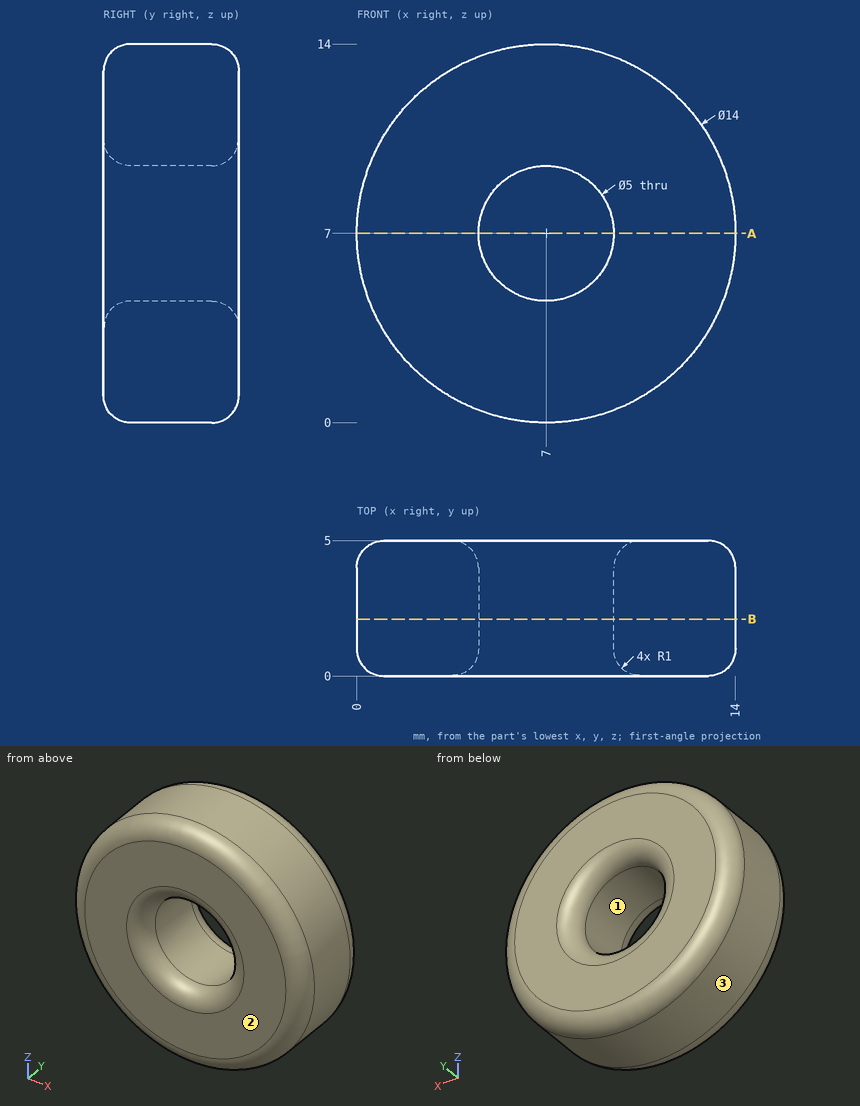
For this review, use the dimensioned drawing (mm, ordinates from the lowest corner) and the shaded views. Give positions to 0.01 mm unless a question says otherwise; leave off trailing zeros. Order: outer loops, then holes, each group sorted by start corner. A loop starts at its lowest first (then second) coordinate and runs counter-clockwise, first axis right, second up.
1) Take a section at A-A (z = 7). Give the boundary of the cut face in (x, y).
2) Wall thickness on line 1 (Z direction, x = 7, y = 2.6); line 2 (Z direction, x = 8, y = 3.75): over which ranges is each line inside the solid? List them lowest first.
3) Insertion check: pin 1 (6.5 mm diameter, centred on x = 7, z = 7, fed in from -Y); pin 2 (1.5 mm diameter, centred on x = 1.5, y = 4, fed in from -Z); pin 3 (3 mm diameter, centred on x = 8.5, y = 3, fed in from -Z); pin 4 (3 mm diameter, centred on x = 9.5, y = 2, fed in from +Z). Each pin has a flat end and moves straight along its axis. Give the tip position at first contact, or say it passes through.
4) Take a section at B-B (y = 2.1). Give the boundary of the cut face in (x, z), then the cut area to 3 significant figures.
5) The part is to be moulded in two halves that separate along X. For the marked faces 1, 2 and 3, say which applies: released by +X, released by -X, zero draft, split by the parting line, or undercut.
Derived:
1. outline: (0, 1) arc R1 ccw to (1, 0) - (3.5, 0) arc R1 ccw to (4.5, 1) - (4.5, 4) arc R1 ccw to (3.5, 5) - (1, 5) arc R1 ccw to (0, 4) - close; (9.5, 1) arc R1 ccw to (10.5, 0) - (13, 0) arc R1 ccw to (14, 1) - (14, 4) arc R1 ccw to (13, 5) - (10.5, 5) arc R1 ccw to (9.5, 4) - close
2. line 1: z = 0 to 4.5, 9.5 to 14
2. line 2: z = 0.07 to 4.71, 9.29 to 13.93
3. pin 1: stops at y = 0.03
3. pin 2: stops at z = 1.86
3. pin 3: stops at z = 0
3. pin 4: stops at z = 13.93
4. outline: circle Ø14 at (7, 7); hole circle Ø5 at (7, 7)
4. area: 134 mm2
5. face 1: undercut
5. face 2: zero draft
5. face 3: split by the parting line
